```python
from build123d import *

# Parameters (mm, degrees)
SKETCH1_W               = 44
SKETCH1_H               = 30
POD_BODY_DEPTH          = 12
SKETCH2_W               = 21.2
SKETCH2_H               = 18.2
BOARD_POCKET_DEPTH      = 5
SKETCH3_R               = 1.1
BOARD_PILOT_HOLES_DEPTH = 9
SKETCH4_R               = 1.1
LID_PILOT_HOLES_DEPTH   = 8
SKETCH5_W               = 12.65
SKETCH5_H               = 8
CABLE_EXIT_DEPTH        = 3.5
STRAP_SLOTS_DEPTH       = 30.206163733
STRAP_SLOTS_DEPTH_BACK  = 30.206163733
SKETCH7_W               = 6
SKETCH7_H               = 3.5


with BuildPart() as part:
    # Sketch1 → Pod Body (new body)
    with BuildSketch(Plane(origin=(0, 0, 0), x_dir=(1, 0, 0), z_dir=(0, 1, 0))):
        Rectangle(SKETCH1_W, SKETCH1_H)
    extrude(amount=POD_BODY_DEPTH)

    # Sketch2 → Board Pocket (cut)
    with BuildSketch(Plane(origin=(0, 12, 0), x_dir=(1, 0, 0), z_dir=(0, 1, 0))):
        Rectangle(SKETCH2_W, SKETCH2_H)
    extrude(amount=-BOARD_POCKET_DEPTH, mode=Mode.SUBTRACT)

    # Sketch3 → Board Pilot Holes (cut)
    with BuildSketch(Plane(origin=(0, 12, 0), x_dir=(1, 0, 0), z_dir=(0, 1, 0))):
        with Locations(Location((-7.6, 5.6, 0), (0, 0, 270))):
            Circle(SKETCH3_R)
        with Locations(Location((7.6, 5.6, 0), (0, 0, 270))):
            Circle(SKETCH3_R)
    extrude(amount=-BOARD_PILOT_HOLES_DEPTH, mode=Mode.SUBTRACT)

    # Sketch4 → Lid Pilot Holes (cut)
    with BuildSketch(Plane(origin=(0, 12, 0), x_dir=(1, 0, 0), z_dir=(0, 1, 0))):
        with Locations(Location((-18, -11, 0), (0, 0, 270))):
            Circle(SKETCH4_R)
        with Locations(Location((-18, 11, 0), (0, 0, 270))):
            Circle(SKETCH4_R)
        with Locations(Location((18, -11, 0), (0, 0, 270))):
            Circle(SKETCH4_R)
        with Locations(Location((18, 11, 0), (0, 0, 270))):
            Circle(SKETCH4_R)
    extrude(amount=-LID_PILOT_HOLES_DEPTH, mode=Mode.SUBTRACT)

    # Sketch5 → Cable Exit (cut)
    with BuildSketch(Plane(origin=(0, 12, 0), x_dir=(1, 0, 0), z_dir=(0, 1, 0))):
        with Locations((16.675, 0)):
            Rectangle(SKETCH5_W, SKETCH5_H)
    extrude(amount=-CABLE_EXIT_DEPTH, mode=Mode.SUBTRACT)

    # Sketch7 → Strap Slots (cut, two sides: drawn at the far end of the back side and taken through both)
    with BuildSketch(Plane.XY.offset(-STRAP_SLOTS_DEPTH_BACK)):
        with Locations((-13, 3.25)):
            Rectangle(SKETCH7_W, SKETCH7_H)
        with Locations((13, 3.25)):
            Rectangle(SKETCH7_W, SKETCH7_H)
    extrude(amount=STRAP_SLOTS_DEPTH + STRAP_SLOTS_DEPTH_BACK, mode=Mode.SUBTRACT)


solid = part.part
```
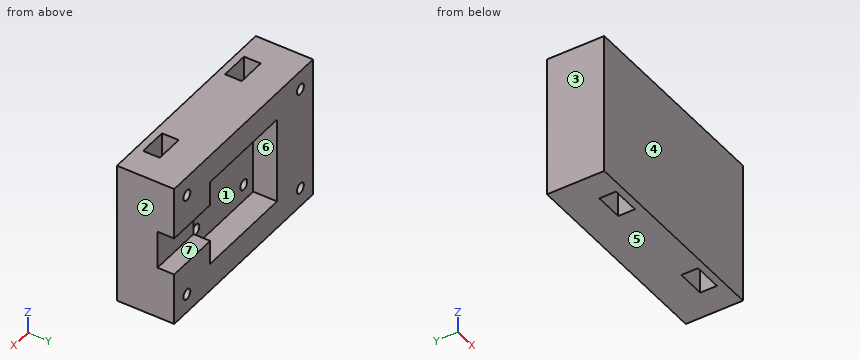
Check sheet for the modelled part. Datum: model origin and axes. Units: mm. Face numbers are marked on the shaded views. A direction names the side the tool comes from. Coordinates: 2 decimals unless noted, no trailing zeros. Write each loop counter-clockwise with the first axis right and the second up, starting at its lowest first coordinate (ties: lowest second). Pieces come first, ordered by that corner, then holes. Notation, with made-up numbers: (70, -20) -> (94, -20) arc R25 cw to (94, -5) -> close; hole circle Ø3 at (82.25, 25). An arc over 180 degrees is marked (long way). Use a Markdown table: item, result.
1. Go/stop test with flat-tipped pins: pin 1 Ø0.7 at (x, z) = (-8, -6) entering from +Y; pin 2 Ø1.1 at (x, z) = (18, 10.5) entering from +Y; pin 3 Ø14.5 at (x, z) = (0, -1) entering from +Y. Record where each tip stops, or that it passes through.
Reported:
| item | result |
|---|---|
| pin 1 | stops at y = 3 |
| pin 2 | stops at y = 4 |
| pin 3 | stops at y = 7 |
2. Scan lines: line 1 along X through (y, z) = (6.2, -5.6); line 2 along X through (y, z) = (9.75, 11); line 3 along Y through (x, z) = (13, 13.5). Record each from-to range of solid material in increasing order.
Reported:
| item | result |
|---|---|
| line 1 | x = -22 to -8.7, -6.5 to 6.5, 8.7 to 22 |
| line 2 | x = -22 to -19.1, -16.9 to 16.9, 19.1 to 22 |
| line 3 | y = 0 to 1.5, 5 to 12 |
3. Sectioned sample at C-C (y = 10). Enter the section's corners in (x, z).
Reported:
| item | result |
|---|---|
| outline | (-22, -15) -> (22, -15) -> (22, -4) -> (10.6, -4) -> (10.6, -9.1) -> (-10.6, -9.1) -> (-10.6, 9.1) -> (10.6, 9.1) -> (10.6, 4) -> (22, 4) -> (22, 15) -> (-22, 15) -> close; hole circle Ø2.2 at (-18, -11); hole circle Ø2.2 at (-18, 11); hole circle Ø2.2 at (18, -11); hole circle Ø2.2 at (18, 11) |
4. Tool access check on the marked faces 5, 6 and 7. Record the directions out of +Z, -Z, +X, -X, +Y, -Y that give a thin tool (end or side, any length) a straight path to the whole face; none if there is none.
Reported:
| item | result |
|---|---|
| face 5 | -Z, +X, -X, +Y, -Y |
| face 6 | +Y |
| face 7 | +X, +Y |
5. Sectioned sample at A-A (x = 11.5). Enter the section's corners in (y, z), plus the area to 3 significant figures.
Reported:
| item | result |
|---|---|
| outline | (0, -15) -> (1.5, -15) -> (1.5, 15) -> (0, 15) -> close; (5, -15) -> (12, -15) -> (12, -4) -> (8.5, -4) -> (8.5, 4) -> (12, 4) -> (12, 15) -> (5, 15) -> close |
| area | 227 mm2 |
6. Sectioned sample at D-D (x = 18). Enter the section's corners in (y, z), plus the area to 3 significant figures.
Reported:
| item | result |
|---|---|
| outline | (0, -15) -> (12, -15) -> (12, -12.1) -> (4, -12.1) -> (4, -9.9) -> (12, -9.9) -> (12, -4) -> (8.5, -4) -> (8.5, 4) -> (12, 4) -> (12, 9.9) -> (4, 9.9) -> (4, 12.1) -> (12, 12.1) -> (12, 15) -> (0, 15) -> close |
| area | 297 mm2 |
7. Sectioned sample at B-B (z = -11). Enter the section's corners in (x, y).
Reported:
| item | result |
|---|---|
| outline | (-22, 0) -> (22, 0) -> (22, 12) -> (19.1, 12) -> (19.1, 4) -> (16.9, 4) -> (16.9, 12) -> (-16.9, 12) -> (-16.9, 4) -> (-19.1, 4) -> (-19.1, 12) -> (-22, 12) -> close; hole (-16, 1.5) -> (-10, 1.5) -> (-10, 5) -> (-16, 5) -> close; hole (10, 1.5) -> (16, 1.5) -> (16, 5) -> (10, 5) -> close |
8. Release check for a two-part mould opening along X. For the marked faces 1, 2, 3 and 4 record: pulls with the +X half, pulls with the -X half, needs draft (parallel to the pull), parting line crosses it, or undercut.
Reported:
| item | result |
|---|---|
| face 1 | undercut |
| face 2 | pulls with the +X half |
| face 3 | pulls with the -X half |
| face 4 | needs draft |
